Geometry check sheet. Reference: drawing and pictorial views, mm from the part's lowest x, y, z. A direction names the side the tool comes from. Give positions to 0.01 mm unless a question says otherwise; leave off trailing zeros. Order: outer loops, then holes, each group sorted by start corner. A loop starts at its lowest first (then second) coordinate and runs counter-clockwise, first axis right, second up.
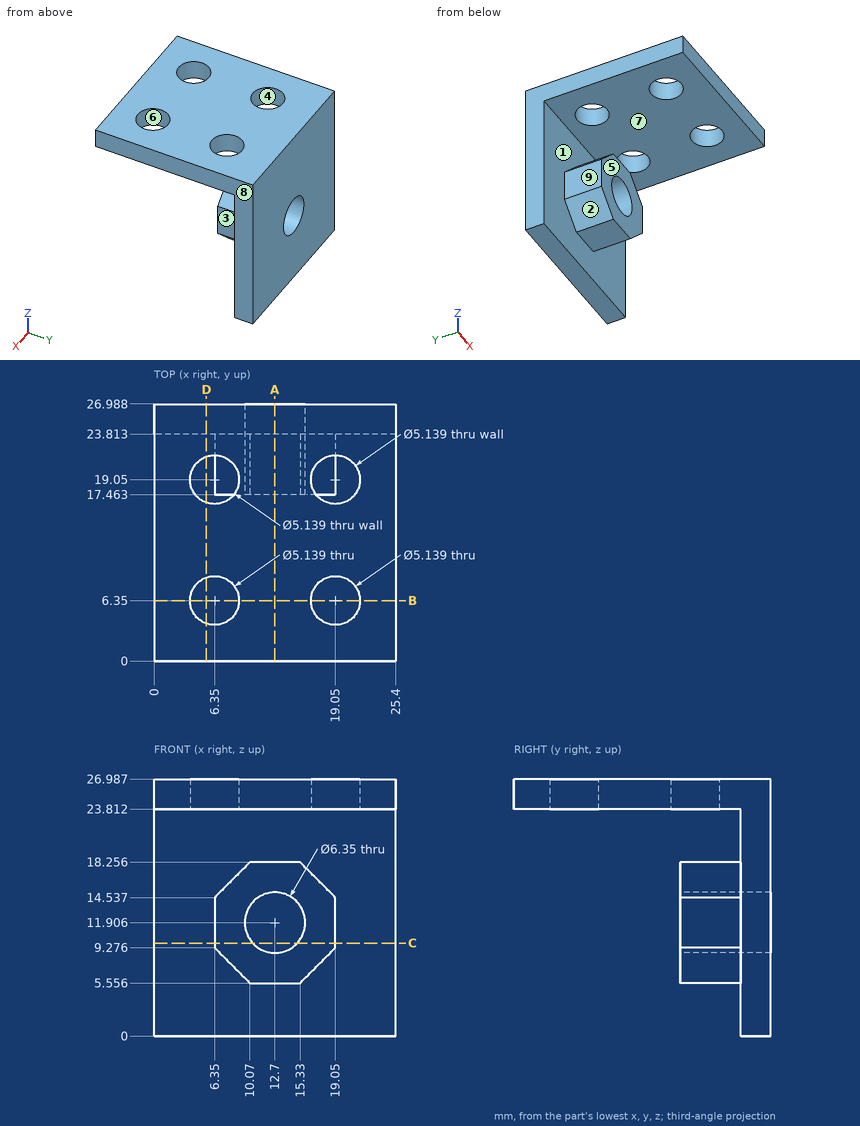
(1) Cross-section at A-A on x = 12.7. Enter the section's corners in (y, z).
Response values:
outline: (0, 23.81) - (23.81, 23.81) - (23.81, 18.26) - (17.46, 18.26) - (17.46, 15.08) - (26.99, 15.08) - (26.99, 26.99) - (0, 26.99) - close; (17.46, 5.56) - (23.81, 5.56) - (23.81, 0) - (26.99, 0) - (26.99, 8.73) - (17.46, 8.73) - close
(2) Cross-section at D-D on x = 5.5. Enter the section's corners in (y, z) (1 decimal).
Response values:
outline: (0, 23.8) - (3.9, 23.8) - (3.9, 27) - (0, 27) - close; (8.8, 23.8) - (16.6, 23.8) - (16.6, 27) - (8.8, 27) - close; (21.5, 23.8) - (23.8, 23.8) - (23.8, 0) - (27, 0) - (27, 27) - (21.5, 27) - close
(3) Gauge pin test, flat ends, axial feed: pin 1 Ø3 at (x, y) = (6.35, 6.35) entering from -Z; pin 2 Ø1.5 at (y, z) = (20, 15.5) entering from +X (1 decimal); pin 3 Ø14 at (x, z) = (13, 9.5) entering from -Y; pin 4 Ø1.5 at (x, z) = (17.5, 21) entering from -Y. Record the tip position at first contact, or that the pin passes through.
Response values:
pin 1: passes through
pin 2: stops at x = 18.8
pin 3: stops at y = 17.46
pin 4: stops at y = 23.81
(4) Release check for a two-part mould opening along X. For the marked faces 6, 7, 8 and 9 record: released by +X, released by -X, zero draft, split by the parting line, or undercut.
Response values:
face 6: undercut
face 7: zero draft
face 8: released by +X
face 9: released by -X
(5) Cross-section at B-B on y = 6.35. Enter the section's corners in (x, z).
Response values:
outline: (0, 23.81) - (3.78, 23.81) - (3.78, 26.99) - (0, 26.99) - close; (8.92, 23.81) - (16.48, 23.81) - (16.48, 26.99) - (8.92, 26.99) - close; (21.62, 23.81) - (25.4, 23.81) - (25.4, 26.99) - (21.62, 26.99) - close
(6) Material ranges on L1, parallel to X at y = 19.05, z = 25.3; L2, parallel to X at y = 17.5, z = 25.75; L3, parallel to Z at x = 9, y = 8.25, recorded low to high.
Response values:
L1: x = 0 to 3.78, 8.92 to 16.48, 21.62 to 25.4
L2: x = 0 to 4.3, 8.4 to 17, 21.1 to 25.4
L3: z = 23.81 to 26.99
(7) Cross-section at C-C on z = 9.75. Enter the section's corners in (x, y), then the cut area to 3 significant figures.
Response values:
outline: (0, 23.81) - (6.35, 23.81) - (6.35, 17.46) - (10.37, 17.46) - (10.37, 26.99) - (0, 26.99) - close; (15.03, 17.46) - (19.05, 17.46) - (19.05, 23.81) - (25.4, 23.81) - (25.4, 26.99) - (15.03, 26.99) - close
area: 117 mm2
(8) Set-up check for the marked faces 1, 2, 3, 4 and 5: record each of +Z, -Z, +X, -X, +Y, -Y from which the full face is reachable in a straight line by a thin tool's end or side.
Response values:
face 1: -Y
face 2: -Z, -X, -Y
face 3: -Z, +X, -Y
face 4: +Z
face 5: -Z, +X, -X, -Y
